Source: CAD feature listing. Evaluate the final solid. Frame: model axes, mm. A direction names the side the tool comes from. Give positions to 0.01 mm unless a question says otherwise; leave off trailing zeros. Loops run counter-clockwise (first coordinate to the right, second up) from the corner with the lowest first, then second, coordinate; pieces in that order, holes last.
from build123d import *

# Parameters (mm, degrees)
EXTRUDE_1_DEPTH             = 115
SKETCH_2_W                  = 66
SKETCH_2_H                  = 5
SKETCH_2_W_2                = 230
SKETCH_2_H_2                = 11.25
SKETCH_2_W_3                = 15.5
SKETCH_2_H_3                = 4
CUT_EXTRUDE_1_DEPTH         = 292.225234599
HOLE_WIZARD_M8_1_D          = 6.8
HOLE_WIZARD_M8_1_DEPTH      = 25
HOLE_WIZARD_M8_1_TIP        = 2.042926105
MM_1_D                      = 8
MM_1_DEPTH                  = 15
MM_1_TIP                    = 2.403442476
HOLE_WIZARD_M5_1_AT_2_COUNT = 2
HOLE_WIZARD_M5_1_AT_2_PITCH = 50


with BuildPart() as part:
    # 草图1 → 凸台-拉伸1 (new, symmetric)
    with BuildSketch(Plane.XY):
        with BuildLine():
            Line((-40.620192023, 87.200904414), (-94, 87.200904414))
            ThreePointArc((-94, 87.200904414), (-97.535533906, 88.665370508), (-99, 92.200904414))
            Line((-99, 92.200904414), (-99, 134.493797632))
            ThreePointArc((-99, 134.493797632), (-99.038060234, 134.685139349), (-99.146446609, 134.847351023))
            Line((-99.146446609, 134.847351023), (-100.853553391, 136.554457804))
            ThreePointArc((-100.853553391, 136.554457804), (-101.015765065, 136.66284418), (-101.207106781, 136.700904414))
            Line((-101.207106781, 136.700904414), (-112.792893219, 136.700904414))
            ThreePointArc((-112.792893219, 136.700904414), (-112.984234935, 136.66284418), (-113.146446609, 136.554457804))
            Line((-113.146446609, 136.554457804), (-114.853553391, 134.847351023))
            ThreePointArc((-114.853553391, 134.847351023), (-114.961939766, 134.685139349), (-115, 134.493797633))
            Line((-115, 134.493797633), (-115, 76.408011195))
            ThreePointArc((-115, 76.408011195), (-114.961939766, 76.216669479), (-114.853553391, 76.054457804))
            Line((-114.853553391, 76.054457804), (-114.146446609, 75.347351023))
            ThreePointArc((-114.146446609, 75.347351023), (-113.984234935, 75.238964647), (-113.792893219, 75.200904414))
            Line((-113.792893219, 75.200904414), (-103.571067812, 75.200904414))
            ThreePointArc((-103.571067812, 75.200904414), (-101.65765065, 74.820302076), (-100.035533906, 73.73643832))
            Line((-100.035533906, 73.73643832), (-94.75, 68.450904414))
            Line((-94.75, 68.450904414), (-79.3, 68.450904414))
            Line((-79.3, 68.450904414), (-76.8, 70.950904414))
            Line((-76.8, 70.950904414), (-65.2, 70.950904414))
            Line((-65.2, 70.950904414), (-62.7, 68.450904414))
            Line((-62.7, 68.450904414), (-50, 68.450904414))
            ThreePointArc((-50, 68.450904414), (-49.646446609, 68.597351023), (-49.5, 68.950904414))
            Line((-49.5, 68.950904414), (-49.5, 69.450904414))
            ThreePointArc((-49.5, 69.450904414), (-45.469068911, 71.427327951), (-46.375, 67.030289822))
            ThreePointArc((-46.375, 67.030289822), (-46.645284708, 66.852353122), (-46.75, 66.546166904))
            Line((-46.75, 66.546166904), (-46.75, 60.450904414))
            ThreePointArc((-46.75, 60.450904414), (-46.457106781, 59.743797632), (-45.75, 59.450904414))
            Line((-45.75, 59.450904414), (-42.286966077, 59.450904414))
            ThreePointArc((-42.286966077, 59.450904414), (-40.609915094, 58.804954035), (-39.799497484, 57.200904414))
            ThreePointArc((-39.799497484, 57.200904414), (-35.270810958, 42.333739964), (-25.417519793, 30.314828464))
            ThreePointArc((-25.417519793, 30.314828464), (-25.268563981, 30.230246377), (-25.099800796, 30.200904414))
            Line((-25.099800796, 30.200904414), (-10.5, 30.200904414))
            ThreePointArc((-10.5, 30.200904414), (-10.146446609, 30.347351023), (-10, 30.700904414))
            Line((-10, 30.700904414), (-10, 43.014370934))
            ThreePointArc((-10, 43.014370934), (-10.066987298, 43.264370934), (-10.25, 43.447383636))
            ThreePointArc((-10.25, 43.447383636), (0, 81.700904414), (10.25, 43.447383636))
            ThreePointArc((10.25, 43.447383636), (10.066987298, 43.264370934), (10, 43.014370934))
            Line((10, 43.014370934), (10, 30.700904414))
            ThreePointArc((10, 30.700904414), (10.146446609, 30.347351023), (10.5, 30.200904414))
            Line((10.5, 30.200904414), (25.099800796, 30.200904414))
            ThreePointArc((25.099800796, 30.200904414), (25.268563981, 30.230246377), (25.417519793, 30.314828464))
            ThreePointArc((25.417519793, 30.314828464), (35.270810958, 42.333739964), (39.799497484, 57.200904414))
            ThreePointArc((39.799497484, 57.200904414), (40.609915094, 58.804954035), (42.286966077, 59.450904414))
            Line((42.286966077, 59.450904414), (45.75, 59.450904414))
            ThreePointArc((45.75, 59.450904414), (46.457106781, 59.743797632), (46.75, 60.450904414))
            Line((46.75, 60.450904414), (46.75, 66.546166904))
            ThreePointArc((46.75, 66.546166904), (46.645284708, 66.852353122), (46.375, 67.030289822))
            ThreePointArc((46.375, 67.030289822), (45.469068911, 71.427327951), (49.5, 69.450904414))
            Line((49.5, 69.450904414), (49.5, 68.950904414))
            ThreePointArc((49.5, 68.950904414), (49.646446609, 68.597351023), (50, 68.450904414))
            Line((50, 68.450904414), (62.7, 68.450904414))
            Line((62.7, 68.450904414), (65.2, 70.950904414))
            Line((65.2, 70.950904414), (76.8, 70.950904414))
            Line((76.8, 70.950904414), (79.3, 68.450904414))
            Line((79.3, 68.450904414), (94.75, 68.450904414))
            Line((94.75, 68.450904414), (100.035533906, 73.73643832))
            ThreePointArc((100.035533906, 73.73643832), (101.65765065, 74.820302076), (103.571067812, 75.200904414))
            Line((103.571067812, 75.200904414), (113.792893219, 75.200904414))
            ThreePointArc((113.792893219, 75.200904414), (113.984234935, 75.238964647), (114.146446609, 75.347351023))
            Line((114.146446609, 75.347351023), (114.853553391, 76.054457804))
            ThreePointArc((114.853553391, 76.054457804), (114.961939766, 76.216669479), (115, 76.408011195))
            Line((115, 76.408011195), (115, 134.493797632))
            ThreePointArc((115, 134.493797632), (114.961939766, 134.685139348), (114.853553391, 134.847351023))
            Line((114.853553391, 134.847351023), (113.146446609, 136.554457804))
            ThreePointArc((113.146446609, 136.554457804), (112.984234935, 136.66284418), (112.792893219, 136.700904414))
            Line((112.792893219, 136.700904414), (101.207106781, 136.700904414))
            ThreePointArc((101.207106781, 136.700904414), (101.015765065, 136.66284418), (100.853553391, 136.554457804))
            Line((100.853553391, 136.554457804), (99.146446609, 134.847351023))
            ThreePointArc((99.146446609, 134.847351023), (99.038060234, 134.685139349), (99, 134.493797632))
            Line((99, 134.493797632), (99, 92.200904414))
            ThreePointArc((99, 92.200904414), (97.535533906, 88.665370508), (94, 87.200904414))
            Line((94, 87.200904414), (40.620192023, 87.200904414))
            ThreePointArc((40.620192023, 87.200904414), (40.56009167, 87.201265632), (40.5, 87.202349235))
            ThreePointArc((40.5, 87.202349235), (39.949738775, 87.246059064), (39.407648979, 87.350158145))
            ThreePointArc((39.407648979, 87.350158145), (19.852534709, 90.98365881), (0, 92.200904414))
            ThreePointArc((0, 92.200904414), (-19.852534708, 90.98365881), (-39.407648978, 87.350158145))
            ThreePointArc((-39.407648978, 87.350158145), (-39.949738774, 87.246059064), (-40.5, 87.202349235))
            ThreePointArc((-40.5, 87.202349235), (-40.56009167, 87.201265632), (-40.620192023, 87.200904414))
        make_face()
    extrude(amount=EXTRUDE_1_DEPTH, both=True)

    # 草图2 → 切除-拉伸1 (cut, through all)
    with BuildSketch(Plane.XY.offset(115)):
        with Locations((-82, 66.950904414)):
            Rectangle(SKETCH_2_W, SKETCH_2_H)
        with Locations((0, 131.075904414)):
            Rectangle(SKETCH_2_W_2, SKETCH_2_H_2)
        with Locations((82, 66.950904414)):
            Rectangle(SKETCH_2_W, SKETCH_2_H)
        with Locations((-107.25, 75.200904414)):
            Rectangle(SKETCH_2_W_3, SKETCH_2_H_3)
        with Locations((107.25, 75.200904414)):
            Rectangle(SKETCH_2_W_3, SKETCH_2_H_3)
    extrude(amount=-CUT_EXTRUDE_1_DEPTH, mode=Mode.SUBTRACT)

    # M8 螺纹孔1
    with Locations(Plane(origin=(0, 125.450904414, 0), x_dir=(1, 0, 0), z_dir=(0, 1, 0))):
        with Locations((-107, 105), (-107, -55), (-107, 55), (-107, -105), (107, 55), (107, -105), (107, 105), (107, -55)):
            Hole(HOLE_WIZARD_M8_1_D / 2, depth=HOLE_WIZARD_M8_1_DEPTH)
            with Locations((0, 0, -(HOLE_WIZARD_M8_1_DEPTH + HOLE_WIZARD_M8_1_TIP / 2))):  # 118° drill point
                Cone(0, HOLE_WIZARD_M8_1_D / 2, HOLE_WIZARD_M8_1_TIP, mode=Mode.SUBTRACT)

    # 大小mm 暗销孔1
    with Locations(Plane(origin=(0, 125.450904414, 0), x_dir=(1, 0, 0), z_dir=(0, 1, 0))):
        with Locations((-107, 0), (107, 0)):
            Hole(MM_1_D / 2, depth=MM_1_DEPTH)
            with Locations((0, 0, -(MM_1_DEPTH + MM_1_TIP / 2))):  # 118° drill point
                Cone(0, MM_1_D / 2, MM_1_TIP, mode=Mode.SUBTRACT)

    # 草图13 → M5 螺纹孔1 (revolve, cut)
    with BuildSketch(Plane(origin=(115, 90.450904414, 25), x_dir=(0, 0, -1), z_dir=(0, 1, 0))):
        Polygon((0, 0), (0, 13.6618073), (2.1, 12.4), (2.1, 0), align=None)
    hole_wizard_m5_1 = revolve(axis=Axis((121.35, 90.450904414, 25), (-1, 0, 0)), mode=Mode.SUBTRACT)

    # M5 螺纹孔1 at 2: M5 螺纹孔1 ×2
    with Locations(*[(0, 0, -i * HOLE_WIZARD_M5_1_AT_2_PITCH) for i in range(1, HOLE_WIZARD_M5_1_AT_2_COUNT)]):
        add(hole_wizard_m5_1, mode=Mode.SUBTRACT)

    # 镜向1: M5 螺纹孔1 across plane
    add(hole_wizard_m5_1.mirror(Plane(origin=(0, 0, 0), x_dir=(0, 0, 1), z_dir=(1, 0, 0))), mode=Mode.SUBTRACT)

    # 镜向1 copy 1 sketch → 镜向1 copy 1 (revolve, cut)
    with BuildSketch(Plane(origin=(-115, 90.450904414, -25), x_dir=(0, 0, -1), z_dir=(0, 1, 0))):
        Polygon((0, 0), (0, -13.6618073), (2.1, -12.4), (2.1, 0), align=None)
    revolve(axis=Axis((-121.35, 90.450904414, -25), (-1, 0, 0)), mode=Mode.SUBTRACT)


solid = part.part
1) Cut plane D-D (x = -29). Return loops of the section in (y, z).
Checks:
outline: (33.65, -115) - (89.59, -115) - (89.59, 115) - (33.65, 115) - close
2) Cut plane A-A (y = 114). State how many separate pieces and enclosed holes the cut face has, and give its area (3 significant figures).
Checks:
separate pieces: 2
enclosed holes: 10
area: 6,970 mm2
3) Ray query, probe 1 along Z at (x, y) = (-107, 106.5); probe 2 along Z at (x, y) = (107, 120.25); probe 3 along Y at (x, z) = (-110, -25). Return the intervals inside material, ascending.
Checks:
probe 1: z = -115 to -108.4, -101.6 to -58.4, -51.6 to 51.6, 58.4 to 101.6, 108.4 to 115
probe 2: z = -115 to -108.4, -101.6 to -58.4, -51.6 to -4, 4 to 51.6, 58.4 to 101.6, 108.4 to 115
probe 3: y = 77.2 to 88.35, 92.55 to 125.45
4) Reachability of faces 1 (the flat face through (107, 77.201, 2)), 2 (the flat face through (71, 70.951, 2)), 3 (the cylindrical face through (-103.6, 112.8, -105.1)), 4 (the flat face through (-87, 69.451, 2)), 5 (the flat face through (68, 87.201, 2)) from +Z, -Z, +X, -X, +Y, -Y: full face, straight path, thin tool, end or side. Return the list, or none.
Checks:
face 1: +Z, -Z, +X, -Y
face 2: +Z, -Z, -Y
face 3: +Y
face 4: +Z, -Z, -X, -Y
face 5: +Z, -Z, +Y
5) Contact query for flat-ended pins moving along their axis: P1, Ø12, axis at x = -14, z = 35, coming from the +Y side; P2, Ø6, axis at y = 36, z = 29, coming from the +X side; P3, Ø1, axis at x = 44, z = 8.5, coming from the -Y side. Output: stop coordinate, or through.
Checks:
P1: stops at y = 92
P2: stops at x = 33.27
P3: stops at y = 59.45
6) Cut plane B-B (x = 15.5). Return loops of the section in (y, z).
Checks:
outline: (30.2, -115) - (47.78, -115) - (47.78, 115) - (30.2, 115) - close; (74.62, -115) - (91.46, -115) - (91.46, 115) - (74.62, 115) - close
7) Cut plane C-C (x = 70.5). Return loops of the section in (y, z).
Checks:
outline: (70.95, -115) - (87.2, -115) - (87.2, 115) - (70.95, 115) - close
8) Pull-direction query (X, two-part tool) for faces 6 (the conical face through (-107.128, 98.763, -54.424)), 7 (the flat face through (-9, 82, -115)), 8 (the flat face through (-99, 109, 2)), 9 (the flat face through (115, 101, 2)); classes: released by +X, released by -X, zero draft, split by the parting line, or undercut.
Checks:
face 6: undercut
face 7: zero draft
face 8: undercut
face 9: released by +X
